Read the model definition and answer for the solid it produces. Units are mm, in the model's axes. Face numbers are marked on the shaded views. Give positions to 0.01 mm unless a question says otherwise; leave off trailing zeros. Order: outer loops, then holes, each group sorted by start corner. A loop starts at its lowest first (then second) coordinate and runs counter-clockwise, first axis right, second up. Notation, with made-up numbers: M -34.75,38 L 23.25,38 A18 ccw 23.25,44 Z; hole C 18.25,-29 d4. An arc over 180 degrees is marked long. Write item = value, one per line. Start each with the question number.
Autodesk Inventor part; units mm, degrees
ref_plane "YZ Plane" through (0, 0, 0) normal (1, 0, 0) x (0, 1, 0)
ref_plane "XZ Plane" through (0, 0, 0) normal (0, 1, 0) x (-1, 0, 0)
ref_plane "XY Plane" through (0, 0, 0) normal (0, 0, 1) x (1, 0, 0)
sketch "Sketch1" plane through (0, 0, 0) normal (0, 1, 0) x (-1, 0, 0)
  line L0 (30, 18.75) -> (-10, 18.75)
  line L1 (30, 18.75) -> (30, -37.25)
  line L2 (-10, 18.75) -> (-10, -37.25)
  line L3 (-10, -37.25) -> (30, -37.25)
  circle A0 centre (5.5, 3.25) radius 10.5
  circle A1 centre (14.5, -21.75) radius 10.5
  point P0 (0, 0)
  dimension "szerokosc_jakas" = 40
  dimension "dlugosc_docisku" = 56
  dimension "srendica_walka" = 21
  dimension "odsuniecie_walka" = 15.5
  dimension "d4" = 15.5
  dimension "d5" = 21
  dimension "przesuniecie_wzgledne_walkow" = 9
  dimension "d7" = 25
extrude "Extrusion1" add sketch "Sketch1" along normal blind 20
sketch "Sketch2" plane through (10, 0, 18.75) normal (1, 0, 0) x (0, 0, -1)
  circle A0 centre (48, 10) radius 4
  line L0 (56, 0) -> (56, 20)
  line L1 (0, 20) -> (56, 20) construction
  circle A1 centre (36, 10) radius 4
  line L2 (69, 10) -> (-3, 10) construction
  point P0 (18.75, 0)
  dimension "d10" = 8
  dimension "d11" = 8
  dimension "d15" = 12
  dimension "d25" = 10
extrude "Extrusion2" cut sketch "Sketch2" against normal blind 10
sketch "Sketch3" plane through (-30, 0, -37.25) normal (-1, 0, 0) x (0, 0, 1)
  circle A0 centre (48, 10) radius 4
  circle A1 centre (36, 10) radius 4
  line L0 (56, 0) -> (56, 20)
  line L1 (0, 0) -> (56, 0)
  line L2 (75, 10) -> (-12, 10) construction
  point P0 (37.25, 0)
  dimension "d18" = 8
  dimension "d19" = 8
  dimension "d21" = 8
  dimension "d22" = 12
  dimension "d24" = 10
extrude "Extrusion3" cut sketch "Sketch3" against normal blind 10
equation "\"szerokosc_jakas\" = szerokosc"
equation "\"dlugosc_docisku\" = dlugosc"
equation "\"srendica_walka\" = srednica_walka"
equation "\"d4\" = -0.5 * przesuniecie_wzgledne_walkow + 0.5 * szerokosc_jakas"
equation "\"d5\" = srednica_walka"
equation "\"d25\" = 0.5 * grubosc"
equation "\"gw\" = glebokosc_gwintu"
equation "\"d24\" = 0.5 * grubosc"
equation "\"d26\" = glebokosc_gwintu"
equation "\"glebokosc_gwintu\" = 10"
equation "\"szerokosc\" = 40"
equation "\"dlugosc\" = 56"
equation "\"srednica_walka\" = 21"
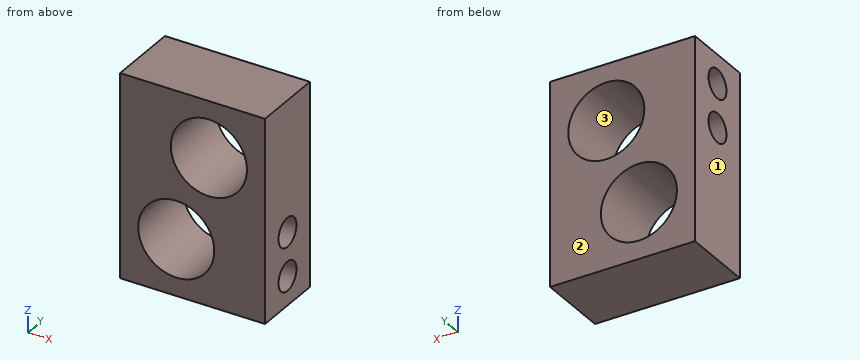
1) Find the intervals of material crossed by probe 1 along Y at (x, z) = (-26.5, -1.25); probe 2 along Z at (x, y) = (-21, 6.5); probe 3 along X at (y, z) = (9.5, 5.5), in increasing order. Write a range as [from, to].
2) Find section B-B on x = -9.5. Determine the outline of the cut face in (y, z), plus the area to 3 significant figures.
3) For a pull along X with two mould halves and no side action, classify the marked faces 1, 2 and 3 as pulls with the +X half, pulls with the -X half, needs draft (parallel to the pull), parting line crosses it, or undercut.
4) Find section D-D on z = -29.25. Determine the outline of the cut face in (x, y), plus the area to 3 significant figures.
5) Find section C-C on y = 10. Determine the outline of the cut face in (x, z), plus the area to 3 significant figures.
6) Find section A-A on z = -1.25. Determine the outline of the cut face in (x, y).
7) Each of these flat-tipped pins is pushed along its axis until it touches: P1, Ø4, axis at y = 9.5, z = -0.5, coming from the -X side; P2, Ø7, axis at y = 10, z = -29.25, coming from the +X side. Where does it stop, or does it pass through?
Numbers:
q1.probe_1 = [0, 6], [14, 20]
q1.probe_2 = [-37.25, -30], [-13.5, -3.19], [0.69, 8.81], [12.69, 18.75]
q1.probe_3 = [-30, -15.76], [4.76, 10]
q2.outline = M 0,-37.25 L 20,-37.25 L 20,-30.98 L 0,-30.98 Z; M 0,-12.52 L 20,-12.52 L 20,-6.46 L 0,-6.46 Z; M 0,12.96 L 20,12.96 L 20,18.75 L 0,18.75 Z
q2.area = 362 mm2
q3.face_1 = pulls with the -X half
q3.face_2 = needs draft
q3.face_3 = undercut
q4.outline = M -30,0 L -21.85,0 L -21.85,20 L -30,20 Z; M -7.15,0 L 10,0 L 10,6 L 0,6 L 0,14 L 10,14 L 10,20 L -7.15,20 Z
q4.area = 426 mm2
q5.outline = M -30,-37.25 L 10,-37.25 L 10,-33.25 L 0,-33.25 L 0,-25.25 L 10,-25.25 L 10,-21.25 L 0,-21.25 L 0,-13.25 L 10,-13.25 L 10,18.75 L -30,18.75 L -30,14.75 L -20,14.75 L -20,6.75 L -30,6.75 L -30,2.75 L -20,2.75 L -20,-5.25 L -30,-5.25 Z; hole C -14.5,-21.75 d21; hole C -5.5,3.25 d21
q5.area = 1,230 mm2
q6.outline = M -30,0 L -14.99,0 L -14.99,20 L -30,20 L -30,14 L -20,14 L -20,6 L -30,6 Z; M 3.99,0 L 10,0 L 10,20 L 3.99,20 Z
q7.P1 = -20
q7.P2 = 0
